Check sheet for the drawn part. Datum: minimum x, y, z corner. Units: mm. A direction names the side the tool comes from. Coordinates: 2 decimals unless noted, no trailing zeros. Write each loop counter-clockwise with the first axis right and the second up, starting at its lowest first coordinate (ties: lowest second). Pieces come first, ordered by that corner, then holes. Notation, with made-up numbers: (35.25, -19) -> (78.25, -19) arc R24 ccw to (78.25, -5) -> close; hole circle Ø8 at (72.25, -35). An arc over 180 degrees is marked (long way). Write each question's results on one line, items separated by ' | '. Start each with the question number.
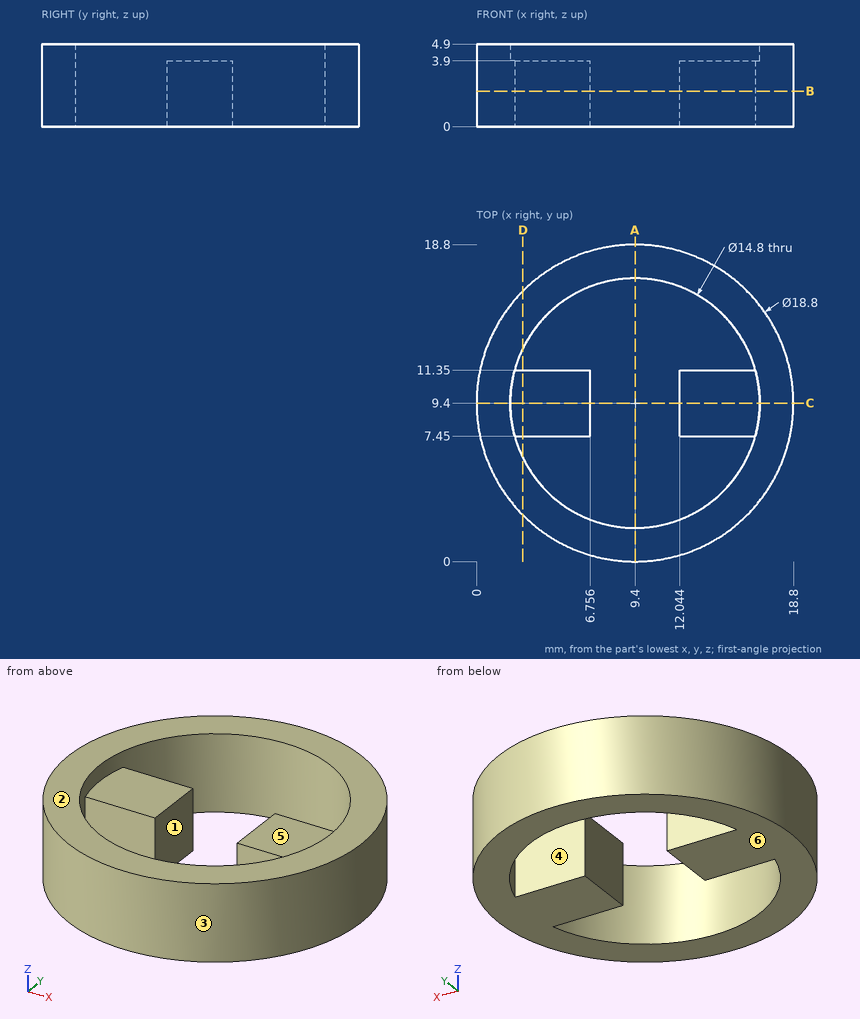
1. Sectioned sample at B-B on z = 2.1. Record the cut outline in (x, y).
2. Sectioned sample at C-C on y = 9.4. Record the cut outline in (x, z).
3. Material ranges on probe 1 along Y at (x, z) = (9.4, 2.9); probe 2 along X at (y, z) = (9.5, 1.7); probe 3 along X at (y, z) = (6.75, 1.7), recorded low to high. Write a range as from..to.
4. Tool access check on the marked faces 4, 5 and 6. Record the directions out of +Z, -Z, +X, -X, +Y, -Y that give a thin tool (end or side, any length) a straight path to the whole face; none if there is none.
5. Depth check by flat-ended pin: pin 1 Ø2 at (x, z) = (5, 2) entering from +Y; pin 2 Ø2 at (y, z) = (12.5, 3) entering from -X; pin 3 Ø1.2 at (x, z) = (4, 1.5) entering from -Y. Enter the tip coordinate at first touch or a pass-through.
6. Sectioned sample at A-A on x = 9.4. Record the cut outline in (y, z).
7. Mould release check, pull along X, two halves, no side actions. Record for the marked faces 1, 2 and 3: +X half, -X half, draft (parallel to the pull), parting line (faces both ways), or undercut.
8. Sectioned sample at D-D on x = 2.75. Record the cut outline in (y, z), plus the area to 3 significant figures.
Computed values:
1) outline: circle Ø18.8 at (9.4, 9.4); hole (2.26, 7.45) arc R7.4 ccw to (16.54, 7.45) -> (12.04, 7.45) -> (12.04, 11.35) -> (16.54, 11.35) arc R7.4 ccw to (2.26, 11.35) -> (6.76, 11.35) -> (6.76, 7.45) -> close
2) outline: (0, 0) -> (6.76, 0) -> (6.76, 3.9) -> (2, 3.9) -> (2, 4.9) -> (0, 4.9) -> close; (12.04, 0) -> (18.8, 0) -> (18.8, 4.9) -> (16.8, 4.9) -> (16.8, 3.9) -> (12.04, 3.9) -> close
3) probe 1: y = 0..2, 16.8..18.8 | probe 2: x = 0..6.76, 12.04..18.8 | probe 3: x = 0.38..2.49, 16.31..18.42
4) face 4: +Z, -Z | face 5: +Z | face 6: -Z, +X, -X, +Y, -Y
5) pin 1: stops at y = 18.16 | pin 2: stops at x = 0.24 | pin 3: stops at y = 1.32
6) outline: (0, 0) -> (2, 0) -> (2, 4.9) -> (0, 4.9) -> close; (16.8, 0) -> (18.8, 0) -> (18.8, 4.9) -> (16.8, 4.9) -> close
7) face 1: undercut | face 2: draft | face 3: parting line
8) outline: (2.76, 0) -> (6.15, 0) -> (6.15, 4.9) -> (2.76, 4.9) -> close; (7.45, 0) -> (11.35, 0) -> (11.35, 3.9) -> (7.45, 3.9) -> close; (12.65, 0) -> (16.04, 0) -> (16.04, 4.9) -> (12.65, 4.9) -> close | area: 48.5 mm^2
